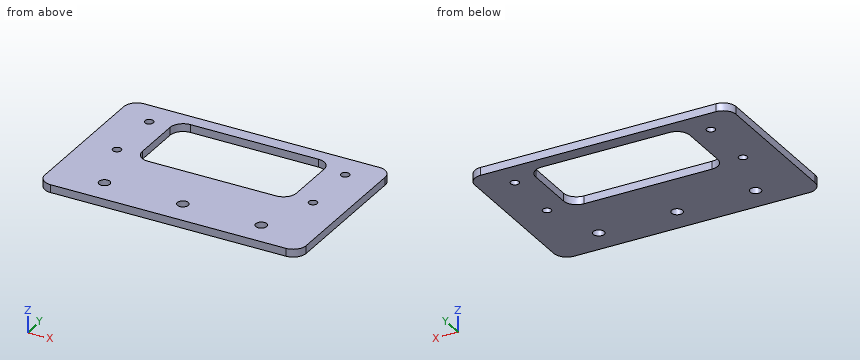
```python
from build123d import *

# Parameters (mm, degrees)
SKETCH_1_W          = 100
SKETCH_1_H          = 64
SKETCH_1_R          = 1.6
SKETCH_1_R_2        = 2.1
EXTRUDE_1_DEPTH     = 3
SKETCH_2_W          = 59
SKETCH_2_H          = 29
CUT_EXTRUDE_1_DEPTH = 10
FILLET_1_R          = 5
FILLET_2_R          = 5


with BuildPart() as part:
    # 草图1 → 凸台-拉伸1 (new body)
    with BuildSketch(Plane.XY):
        Rectangle(SKETCH_1_W, SKETCH_1_H)
        with Locations((-37.5, 0)):
            Circle(SKETCH_1_R, mode=Mode.SUBTRACT)
        with Locations((-37.5, 22)):
            Circle(SKETCH_1_R, mode=Mode.SUBTRACT)
        with Locations((37.5, 0)):
            Circle(SKETCH_1_R, mode=Mode.SUBTRACT)
        with Locations((37.5, 22)):
            Circle(SKETCH_1_R, mode=Mode.SUBTRACT)
        with Locations((-30, -22)):
            Circle(SKETCH_1_R_2, mode=Mode.SUBTRACT)
        with Locations((30, -22)):
            Circle(SKETCH_1_R_2, mode=Mode.SUBTRACT)
        with Locations((0, -22)):
            Circle(SKETCH_1_R_2, mode=Mode.SUBTRACT)
    extrude(amount=EXTRUDE_1_DEPTH)

    # 草图2 → 切除-拉伸1 (cut)
    with BuildSketch(Plane.XY.offset(3)):
        with Locations((0, 12.5)):
            Rectangle(SKETCH_2_W, SKETCH_2_H)
    extrude(amount=-CUT_EXTRUDE_1_DEPTH, mode=Mode.SUBTRACT)

    # 圆角1
    fillet_1_edges = [part.edges().sort_by_distance(p)[0] for p in [
        (29.5, 27, 1.5),
        (29.5, -2, 1.5),
        (-29.5, -2, 1.5),
        (-29.5, 27, 1.5),
    ]]
    fillet(fillet_1_edges, radius=FILLET_1_R)

    # 圆角2
    fillet_2_edges = [part.edges().sort_by_distance(p)[0] for p in [
        (50, -32, 1.5),
        (-50, -32, 1.5),
        (-50, 32, 1.5),
        (50, 32, 1.5),
    ]]
    fillet(fillet_2_edges, radius=FILLET_2_R)


solid = part.part
```
Geometry: final body of the model. Coordinates: model frame, mm. Coordinates: 2 decimals unless noted, no trailing zeros. Order: outer loops, then holes, each group sorted by start corner. A loop starts at its lowest first (then second) coordinate and runs counter-clockwise, first axis right, second up.
Item 1: Material intervals for line 1 along Y through (x, z) = (-37.5, 2.2); line 2 along Y through (x, z) = (0, 1.4); line 3 along Y through (x, z) = (-17, 0.25), sorted ascending.
Answer:
line 1: y = -32 to -1.6, 1.6 to 20.4, 23.6 to 32
line 2: y = -32 to -24.1, -19.9 to -2, 27 to 32
line 3: y = -32 to -2, 27 to 32
Item 2: Contact query for a flat-ended pin moving along its axis: P1, Ø3, axis at x = 37.5, y = 0, coming from the -Z side. Output: stop coordinate, or through.
Answer:
P1: passes through
Item 3: Section query D-D (x = 0). Output: boundary loops of the cut face in (y, z).
Answer:
outline: (-32, 0) - (-24.1, 0) - (-24.1, 3) - (-32, 3) - close; (-19.9, 0) - (-2, 0) - (-2, 3) - (-19.9, 3) - close; (27, 0) - (32, 0) - (32, 3) - (27, 3) - close
Item 4: Section query C-C (z = 1.95). State how many separate pieces and enclosed holes the cut face has, then the cut area to 3 significant figures.
Answer:
separate pieces: 1
enclosed holes: 8
area: 4,620 mm2
Item 5: Section query A-A (x = -17). Output: boundary loops of the cut face in (y, z).
Answer:
outline: (-32, 0) - (-2, 0) - (-2, 3) - (-32, 3) - close; (27, 0) - (32, 0) - (32, 3) - (27, 3) - close
Item 6: Section query B-B (y = 0). Output: boundary loops of the cut face in (x, z), then the cut area to 3 significant figures.
Answer:
outline: (-50, 0) - (-39.1, 0) - (-39.1, 3) - (-50, 3) - close; (-35.9, 0) - (-28.5, 0) - (-28.5, 3) - (-35.9, 3) - close; (28.5, 0) - (35.9, 0) - (35.9, 3) - (28.5, 3) - close; (39.1, 0) - (50, 0) - (50, 3) - (39.1, 3) - close
area: 110 mm2
